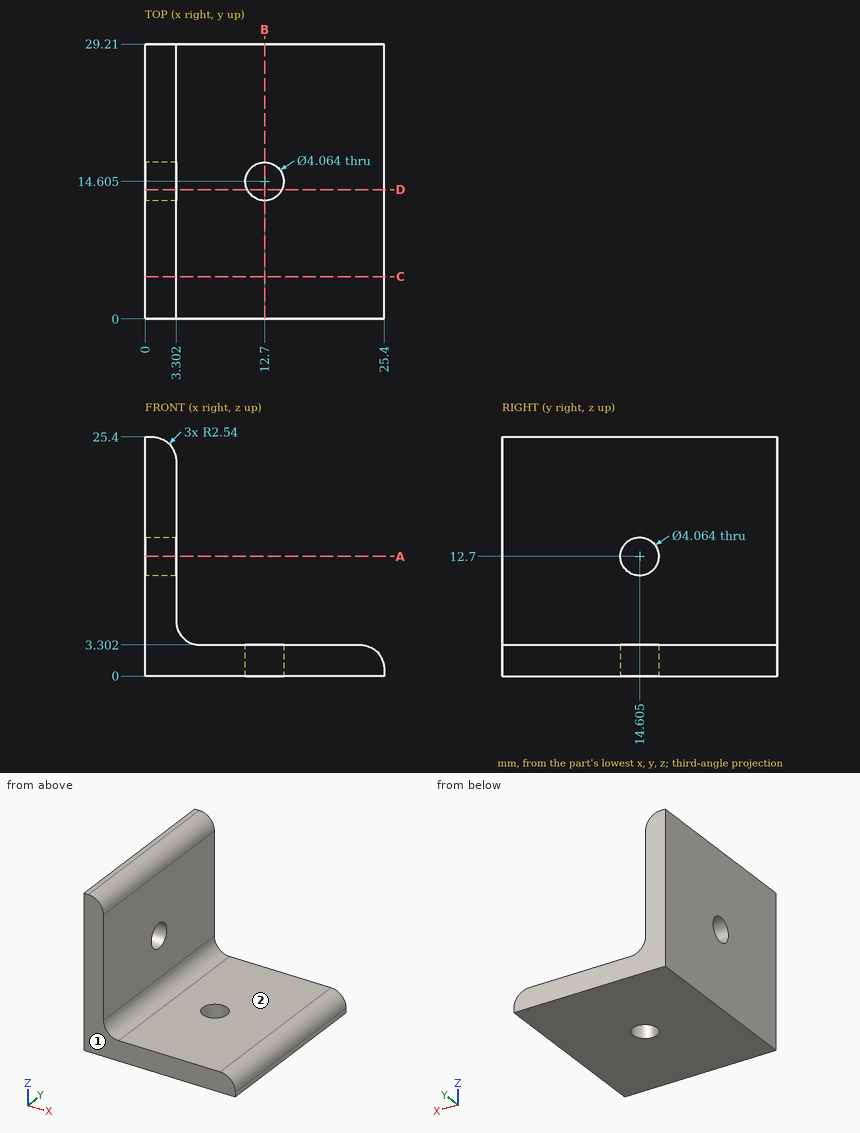
The figure shows three views and two pictorial views of one solid part (mm, origin at its lowest corner). Answer the questions. A direction names the side the tool comes from. Coordinates: 2 decimals unless noted, no trailing zeros. Order: outer loops, then holes, each group sorted by start corner. A loop starts at its lowest first (then second) coordinate and runs counter-clockwise, first axis right, second up. Notation, with made-up numbers: M -23,43 L 23,43 A31 cw 23,78 Z; hole C -20,50 d7. An arc over 180 degrees is marked long. Use CSV: the item, a comma, the result in double quotes.
1) Flat-ended cylindrical pins translate along their axes: pin 1 Ø10 at (y, z) = (10, 6) entering from +X; pin 2 Ø12 at (y, z) = (16.5, 20.5) entering from +X; pin 3 Ø5 at (x, y) = (13.5, 23) entering from +Z. Find the tip coordinate at first contact, or state that the pin passes through.
Worked out:
pin 1,"stops at x = 25.39"
pin 2,"stops at x = 3.3"
pin 3,"stops at z = 3.3"
2) For the marked faces 1 and 2, determine the directions among +Z, -Z, +X, -X, +Y, -Y from which every point of the face is accessible in a straight line to the end or side of a thin tool.
Worked out:
face 1,"+Z, -Z, +X, -X, -Y"
face 2,"+Z, +X, +Y, -Y"
3) Section D-D on y = 13.75 is taken. Write down the section's boundary in (x, z), plus the area to 3 significant figures.
Worked out:
outline,"M 0,0 L 10.86,0 L 10.86,3.3 L 5.84,3.3 A2.54 cw 3.3,5.84 L 3.3,10.86 L 0,10.86 Z; M 0,14.54 L 3.3,14.54 L 3.3,22.86 A2.54 ccw 0.76,25.4 L 0,25.4 Z; M 14.54,0 L 25.4,0 L 25.4,0.76 A2.54 ccw 22.86,3.3 L 14.54,3.3 Z"
area,"131 mm^2"
4) Consider line 1 (Y direction, x = 12.7, z = 1.35); line 2 (Z direction, x = 21.5, y = 6.25). Determine where each line is inside the solid, lowest interval first. Write a range as [from, to].
Worked out:
line 1,"y = [0, 12.57], [16.64, 29.21]"
line 2,"z = [0, 3.3]"
5) Section B-B on x = 12.7 is taken. Write down the section's boundary in (y, z).
Worked out:
outline,"M 0,0 L 12.57,0 L 12.57,3.3 L 0,3.3 Z; M 16.64,0 L 29.21,0 L 29.21,3.3 L 16.64,3.3 Z"
6) Section C-C on y = 4.5 is taken. Write down the section's boundary in (x, z).
Worked out:
outline,"M 0,0 L 25.4,0 L 25.4,0.76 A2.54 ccw 22.86,3.3 L 5.84,3.3 A2.54 cw 3.3,5.84 L 3.3,22.86 A2.54 ccw 0.76,25.4 L 0,25.4 Z"
7) Section A-A on z = 12.7 is taken. Write down the section's boundary in (x, y), plus the area to 3 significant figures.
Worked out:
outline,"M 0,0 L 3.3,0 L 3.3,12.57 L 0,12.57 Z; M 0,16.64 L 3.3,16.64 L 3.3,29.21 L 0,29.21 Z"
area,"83.0 mm^2"
